Here's how the part is built. I have some questions about the finished solid (model axes, mm). Face numbers are marked on the shaded views. A direction names the side the tool comes from. Round coordinates to 2 decimals unless told otherwise and drop trailing zeros. Write each loop counter-clockwise with the first axis right and the second up, starting at its lowest first coordinate (ties: lowest second). Pieces come first, ordered by that corner, then holes. Notation, with made-up numbers: (-30.75, -17) -> (-19.75, -17) arc R26 ccw to (-19.75, -2) -> close; hole circle Ø11 at (78, 65). An arc over 180 degrees is marked (long way). Put each result on its own line as item: value. Start each with the question number.
1) Which directions (+Z, -Z, +X, -X, +Y, -Y) give clear straight access to the entire face, cutting with the end or side of a thin tool? Please do the marked faces 1, 2 and 3.
2) I want a section at C-C, the plane y = -2.2. List the corners of the cut face in (x, z) for me, then the cut area to 3 significant figures.
3) I want a section at B-B, the plane x = -11.2. List the corners of the cut face in (y, z) for me.
4) Will these pins go through, and if not, where does the flat tip stop? P1, Ø1.2, axis at x = -4, z = -1.27, coming from the +Y side; P2, Ø2.5, axis at x = 4, z = 1.27, coming from the +Y side; P3, Ø1.5, axis at y = -1.5, z = -3, coming from the +X side; P4, Ø2, axis at x = 2.5, z = -0.5, coming from the -Y side.
5) We'd pull the mould along Z, two halves only. Please class the marked faces 4, 5 and 6: released by +Z, released by -Z, zero draft, split by the parting line, or undercut.
6) I want a section at A-A, the plane x = -4. List the corners of the cut face in (y, z) for me.
7) If I drill on line 1 along X through (y, z) = (1, 0); line 2 along Z through (x, y) = (-4, -2.95); line 3 along X through (y, z) = (-2.2, -1.27), over which ranges is the centre line in solid material (lowest first)? Write a range as [from, to].
8) I want a section at D-D, the plane z = 3.25. List the corners of the cut face in (x, y) for me.
from build123d import *

# Parameters (mm, degrees)
SKETCH1_W           = 30.4
SKETCH1_H           = 8
SKETCH1_R           = 1.55
SKETCH1_R_2         = 1
BOSS_EXTRUDE1_DEPTH = 2
SKETCH3_W           = 1
SKETCH3_H           = 8
BOSS_EXTRUDE2_DEPTH = 4
BOSS_EXTRUDE3_START = 4
SKETCH4_W           = 7.5
SKETCH4_H           = 8
SKETCH4_R           = 1
BOSS_EXTRUDE3_DEPTH = 4
SKETCH6_W           = 6
SKETCH6_H           = 8
SKETCH6_R           = 1.55
BOSS_EXTRUDE4_DEPTH = 2


with BuildPart() as part:
    # Sketch1 → Boss-Extrude1 (new body)
    with BuildSketch(Plane(origin=(0, 0, 0), x_dir=(1, 0, 0), z_dir=(0, 1, 0))):
        Rectangle(SKETCH1_W, SKETCH1_H)
        with Locations(Location((-11.2, 0, 0), (0, 0, 270))):
            Circle(SKETCH1_R, mode=Mode.SUBTRACT)
        with Locations(Location((11.2, 0, 0), (0, 0, 90))):
            Circle(SKETCH1_R, mode=Mode.SUBTRACT)
        with Locations(Location((-4, 1.27, 0), (0, 0, 270))):
            Circle(SKETCH1_R_2, mode=Mode.SUBTRACT)
        with Locations(Location((-4, -1.27, 0), (0, 0, 270))):
            Circle(SKETCH1_R_2, mode=Mode.SUBTRACT)
        with Locations(Location((4, 1.27, 0), (0, 0, 270))):
            Circle(SKETCH1_R_2, mode=Mode.SUBTRACT)
        with Locations(Location((4, -1.27, 0), (0, 0, 270))):
            Circle(SKETCH1_R_2, mode=Mode.SUBTRACT)
    extrude(amount=BOSS_EXTRUDE1_DEPTH)

    # Sketch3 → Boss-Extrude2 (add)
    with BuildSketch(Plane.XZ):
        Rectangle(SKETCH3_W, SKETCH3_H)
    extrude(amount=BOSS_EXTRUDE2_DEPTH)

    # Sketch4 → Boss-Extrude3 (add)
    with BuildSketch(Plane.XZ.offset(BOSS_EXTRUDE3_START)):
        with Locations((-4.25, 0)):
            Rectangle(SKETCH4_W, SKETCH4_H)
        with Locations(Location((-4, 1.27, 0), (0, 0, 90))):
            Circle(SKETCH4_R, mode=Mode.SUBTRACT)
        with Locations(Location((-4, -1.27, 0), (0, 0, 90))):
            Circle(SKETCH4_R, mode=Mode.SUBTRACT)
    extrude(amount=-BOSS_EXTRUDE3_DEPTH)

    # Sketch6 → Boss-Extrude4 (add)
    # profile 1 of 2: a face of its own
    with BuildSketch(Plane(origin=(0, 2, 0), x_dir=(1, 0, 0), z_dir=(0, 1, 0))):
        with Locations((-18.2, 0)):
            Rectangle(SKETCH6_W, SKETCH6_H)
        with Locations(Location((-17.2, 0.040141274, 0), (0, 0, 270))):
            Circle(SKETCH6_R, mode=Mode.SUBTRACT)
    # profile 2 of 2: a face of its own
    with BuildSketch(Plane(origin=(0, 2, 0), x_dir=(1, 0, 0), z_dir=(0, 1, 0))):
        with Locations((18.2, 0)):
            Rectangle(SKETCH6_W, SKETCH6_H)
        with Locations(Location((17.2, 0.040141274, 0), (0, 0, 270))):
            Circle(SKETCH6_R, mode=Mode.SUBTRACT)
    extrude(amount=-BOSS_EXTRUDE4_DEPTH)


solid = part.part
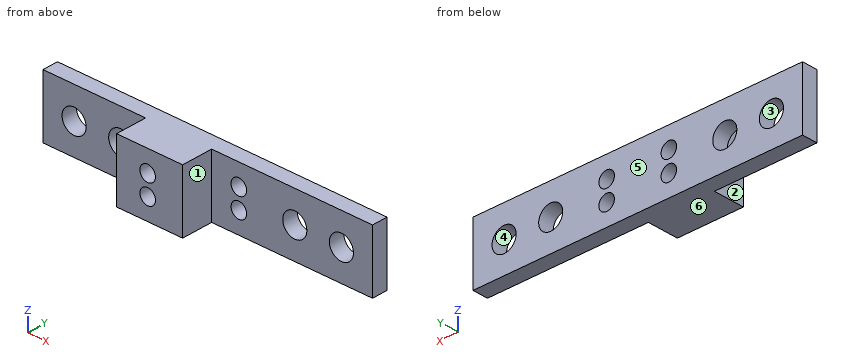
Findings:
1. face 1: +Z, -Z, +X, -Y
1. face 2: +Z, -Z, -X, -Y
1. face 3: +Y, -Y
2. outline: (-8, -4) -> (0.5, -4) -> (0.5, 4) -> (-8, 4) -> close; hole circle Ø2 at (-4, -1.27); hole circle Ø2 at (-4, 1.27)
2. area: 61.7 mm2
3. outline: (0, -4) -> (2, -4) -> (2, -1.55) -> (0, -1.55) -> close; (0, 1.55) -> (2, 1.55) -> (2, 4) -> (0, 4) -> close
4. P1: passes through
4. P2: stops at y = 2
4. P3: stops at x = 0.5
4. P4: stops at y = 0
5. face 4: undercut
5. face 5: zero draft
5. face 6: released by -Z
6. outline: (-4, -4) -> (2, -4) -> (2, -2.27) -> (-4, -2.27) -> close; (-4, -0.27) -> (2, -0.27) -> (2, 0.27) -> (-4, 0.27) -> close; (-4, 2.27) -> (2, 2.27) -> (2, 4) -> (-4, 4) -> close
7. line 1: x = [-21.2, -18.75], [-15.65, -12.75], [-9.65, 9.65], [12.75, 15.65], [18.75, 21.2]
7. line 2: z = [-4, -2.27], [-0.27, 0.27], [2.27, 4]
7. line 3: x = [-8, -5], [-3, 0.5]
8. outline: (-21.2, 0) -> (-8, 0) -> (-8, -4) -> (0.5, -4) -> (0.5, 0) -> (21.2, 0) -> (21.2, 2) -> (-21.2, 2) -> close
